Here's the drawing with two shaded views (mm, measured from the low corner). I have some questions. A direction names the side the tool comes from. Give positions to 0.01 mm unless a question says otherwise; leave off trailing zeros. Order: outer loops, then holes, each group sorted by start corner. A loop starts at its lowest first (then second) coordinate and runs counter-clockwise, first axis right, second up. Notation, with made-up numbers: M 73,86.5 L 100,86.5 A18 cw 100,97.5 Z; hole C -8,24 d1. An arc over 180 degrees is marked long. Write each question's results on one line, items separated by ' | '.
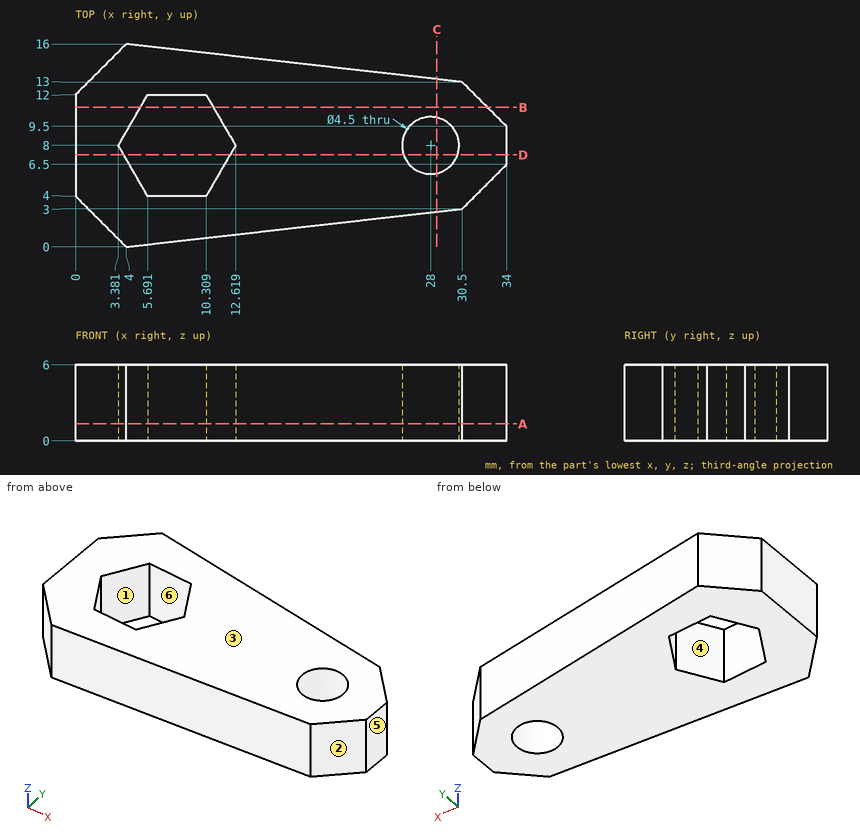
(1) Imagine slicing it at A-A, the plane z = 1.35. Write out the boundary of the cut face in (x, y).
Data:
outline: M 0,4 L 4,0 L 30.5,3 L 34,6.5 L 34,9.5 L 30.5,13 L 4,16 L 0,12 Z; hole M 3.38,8 L 5.69,4 L 10.31,4 L 12.62,8 L 10.31,12 L 5.69,12 Z; hole C 28,8 d4.5
(2) Imagine slicing it at D-D, the plane y = 7.25. Write out the boundary of the cut face in (x, z) (1 decimal), plus the area to 3 significant figures.
Data:
outline: M 0,0 L 3.8,0 L 3.8,6 L 0,6 Z; M 12.2,0 L 25.9,0 L 25.9,6 L 12.2,6 Z; M 30.1,0 L 34,0 L 34,6 L 30.1,6 Z | area: 128 mm2
(3) I need wall thicknesses on L1, parallel to Y at x = 9, z = 2.8; L2, parallel to Y at x = 26, z = 5.4; L3, parallel to X at y = 10.5, z = 2 (1 decimal). Which ranges of each line are inside material? Lowest first, please. Write a range as from..to.
Data:
L1: y = 0.57..4, 12..15.43 | L2: y = 2.49..6.97, 9.03..13.51 | L3: x = 0..4.8, 11.2..33
(4) Imagine slicing it at C-C, the plane x = 28.5. Write out the boundary of the cut face in (y, z), plus the area to 3 significant figures.
Data:
outline: M 2.77,0 L 5.81,0 L 5.81,6 L 2.77,6 Z; M 10.19,0 L 13.23,0 L 13.23,6 L 10.19,6 Z | area: 36.4 mm2
(5) We'd pull the mould along X, two halves only. Please class the marked faces 1, 2, 3 and 4: +X half, -X half, draft (parallel to the pull), parting line (faces both ways), or undercut.
Data:
face 1: undercut | face 2: +X half | face 3: draft | face 4: undercut
(6) Imagine slicing it at B-B, the plane y = 11. Write out the boundary of the cut face in (x, z), plus the area to 3 significant figures.
Data:
outline: M 0,0 L 5.11,0 L 5.11,6 L 0,6 Z; M 10.89,0 L 32.5,0 L 32.5,6 L 10.89,6 Z | area: 160 mm2
(7) For the marked faces 5 and 6, which set-ups out of +Z, -Z, +X, -X, +Y, -Y let a thin tool reach every point of the face, with its end or its side?
Data:
face 5: +Z, -Z, +X, +Y, -Y | face 6: +Z, -Z
